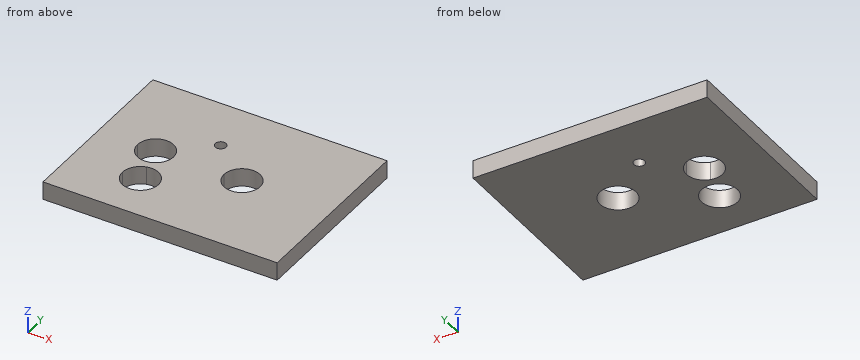
```python
from build123d import *

# Parameters (mm, degrees)
SKETCH3_W           = 65
SKETCH3_H           = 50
BOSS_EXTRUDE2_DEPTH = 5
SKETCH4_R           = 1.5
CUT_EXTRUDE2_DEPTH  = 5
CUT_EXTRUDE3_START  = -10
CUT_EXTRUDE3_DEPTH  = 10


with BuildPart() as part:
    # Sketch3 → Boss-Extrude2 (new body)
    with BuildSketch(Plane.XY):
        with Locations((32.5, -25)):
            Rectangle(SKETCH3_W, SKETCH3_H)
    extrude(amount=BOSS_EXTRUDE2_DEPTH)

    # Sketch4 → Cut-Extrude2 (cut)
    with BuildSketch(Plane.XY.offset(5)):
        with Locations((40, -25)):
            Circle(SKETCH4_R)
        with Locations((16, -25)):
            Circle(SKETCH4_R)
        with Locations((27.986991667, -15.016411928)):
            Circle(SKETCH4_R)
    extrude(amount=-CUT_EXTRUDE2_DEPTH, mode=Mode.SUBTRACT)

    # Sketch5 → Cut-Extrude3 (cut)
    with BuildSketch(Plane(origin=(0, 0, 0), x_dir=(-1, 0, 0), z_dir=(0, 0, -1)).offset(CUT_EXTRUDE3_START)):
        with BuildLine():
            ThreePointArc((-38.689834025, -25.730386964), (-41.451765987, -24.622673194), (-38.5, -25))
            Line((-38.5, -25), (-35, -25))
            ThreePointArc((-35, -25), (-44.839219957, -23.742243979), (-35.632780083, -27.434623214))
            Line((-35.632780083, -27.434623214), (-38.689834025, -25.730386964))
        make_face()
        with BuildLine():
            Line((-35, -25), (-38.5, -25))
            ThreePointArc((-38.5, -25), (-38.548234013, -25.377326806), (-38.689834025, -25.730386964))
            Line((-38.689834025, -25.730386964), (-35.632780083, -27.434623214))
            ThreePointArc((-35.632780083, -27.434623214), (-35.160780043, -26.257756021), (-35, -25))
        make_face()
        with BuildLine():
            ThreePointArc((-17.730991736, -31.885758318), (-20.933750127, -32.145250419), (-23.317219917, -34.300260679))
            Line((-23.317219917, -34.300260679), (-18.95, -36.734883894))
            Line((-18.95, -36.734883894), (-17.730991736, -31.885758318))
        make_face()
        with BuildLine():
            Line((-18.95, -36.734883894), (-23.317219917, -34.300260679))
            ThreePointArc((-23.317219917, -34.300260679), (-20.207756021, -41.574103851), (-13.95, -36.734883894))
            ThreePointArc((-13.95, -36.734883894), (-15.006965552, -33.660395426), (-17.730991736, -31.885758318))
            Line((-17.730991736, -31.885758318), (-18.95, -36.734883894))
        make_face()
        with BuildLine():
            ThreePointArc((-11, -25), (-16, -20), (-21, -25))
            Line((-21, -25), (-17.5, -25))
            ThreePointArc((-17.5, -25), (-16, -23.5), (-14.5, -25))
            ThreePointArc((-14.5, -25), (-15.07765346, -26.182910335), (-16.365702479, -26.454737673))
            Line((-16.365702479, -26.454737673), (-17.219008264, -29.849125576))
            ThreePointArc((-17.219008264, -29.849125576), (-12.925511532, -28.943034448), (-11, -25))
        make_face()
        with BuildLine():
            Line((-17.5, -25), (-21, -25))
            ThreePointArc((-21, -25), (-19.943034448, -28.074488468), (-17.219008264, -29.849125576))
            Line((-17.219008264, -29.849125576), (-16.365702479, -26.454737673))
            ThreePointArc((-16.365702479, -26.454737673), (-17.182910335, -25.92234654), (-17.5, -25))
        make_face()
    extrude(amount=CUT_EXTRUDE3_DEPTH, mode=Mode.SUBTRACT)


solid = part.part
```
Geometry check sheet. Reference: the model listing, model coordinates, mm. Coordinates: 2 decimals unless noted, no trailing zeros. Order: outer loops, then holes, each group sorted by start corner. A loop starts at its lowest first (then second) coordinate and runs counter-clockwise, first axis right, second up. Notation, with made-up numbers: (44, 61.25) - (64, 61.25) arc R21 cw to (64, 93.25) - close; hole circle Ø10 at (-12.75, 65). An arc over 180 degrees is marked (long way). Answer in a Markdown table with one row per item. Add a question column.
1. Gauge pin test, flat ends, axial feed: pin 1 Ø1.5 at (x, y) = (39.5, -40.5) entering from -Z; pin 2 Ø9 at (x, y) = (40, -25) entering from +Z. Record the tip position at first contact, or that the pin passes through.
2. Section check D-D (z = 0.75). Enter the section's corners in (x, y), plus the area to 3 significant figures.
3. Section check A-A (x = 43). Enter the section's corners in (y, z), plus the area to 3 significant figures.
4. Material ranges on L1, parallel to X at y = -25, z = 3.55; L2, parallel to Y at x = 19, z = 1.05; L3, parallel to X at y = -29.5, z = 4.05, recorded low to high. Write a range as [from, to].
5. Section check B-B (x = 16). Enter the section's corners in (y, z), plus the area to 3 significant figures.
6. Section check C-C (y = -35.5). Enter the section's corners in (x, z), plus the area to 3 significant figures.
Data:
| question | item | result |
|---|---|---|
| 1 | pin 1 | stops at z = 0 |
| 1 | pin 2 | passes through |
| 2 | outline | (0, -50) - (65, -50) - (65, 0) - (0, 0) - close; hole circle Ø10 at (16, -25); hole circle Ø10 at (18.95, -36.73); hole circle Ø3 at (27.99, -15.02); hole circle Ø10 at (40, -25) |
| 2 | area | 3,010 mm² |
| 3 | outline | (-50, 0) - (-29, 0) - (-29, 5) - (-50, 5) - close; (-21, 0) - (0, 0) - (0, 5) - (-21, 5) - close |
| 3 | area | 210 mm² |
| 4 | L1 | x = [0, 11], [21, 35], [45, 65] |
| 4 | L2 | y = [-50, -41.73], [-31.74, -29], [-21, 0] |
| 4 | L3 | x = [0, 13.82], [18.18, 37.82], [42.18, 65] |
| 5 | outline | (-50, 0) - (-40.77, 0) - (-40.77, 5) - (-50, 5) - close; (-32.7, 0) - (-30, 0) - (-30, 5) - (-32.7, 5) - close; (-20, 0) - (0, 0) - (0, 5) - (-20, 5) - close |
| 5 | area | 160 mm² |
| 6 | outline | (0, 0) - (14.1, 0) - (14.1, 5) - (0, 5) - close; (23.8, 0) - (65, 0) - (65, 5) - (23.8, 5) - close |
| 6 | area | 277 mm² |
